For this review, take the finished solid that the model builds, in its own axes (mm). A direction names the side the tool comes from. Round coordinates to 2 decimals unless told otherwise and drop trailing zeros. Order: outer loops, then holes, each group sorted by start corner. A loop starts at its lowest first (then second) coordinate and runs counter-clockwise, first axis right, second up. Notation, with made-up numbers: (36, -18.75) -> (62, -18.75) arc R32 ccw to (62, 9.25) -> close; hole circle Ø3 at (-18, -23.75). An arc over 180 degrees is marked (long way). Answer in a Markdown table with one row per item.
```python
from build123d import *

# Parameters (mm, degrees)
SKETCH1_W           = 55
SKETCH1_H           = 67
BOSS_EXTRUDE1_DEPTH = 60
SKETCH3_W           = 8
SKETCH3_H           = 17.5
CUT_EXTRUDE3_DEPTH  = 58
SKETCH4_W           = 4
SKETCH4_H           = 1
SKETCH4_W_2         = 2.5
SKETCH4_H_2         = 15.5
SKETCH4_W_3         = 8
BOSS_EXTRUDE2_DEPTH = 2


with BuildPart() as part:
    # Sketch1 → Boss-Extrude1 (new body)
    with BuildSketch(Plane(origin=(0, 0, 0), x_dir=(1, 0, 0), z_dir=(0, 1, 0))):
        Rectangle(SKETCH1_W, SKETCH1_H)
    extrude(amount=BOSS_EXTRUDE1_DEPTH)

    # Sketch3 → Cut-Extrude3 (cut)
    with BuildSketch(Plane(origin=(0, 60, 0), x_dir=(1, 0, 0), z_dir=(0, 1, 0))):
        Polygon((-18, 13.5), (-18, 31), (-4, 31), (-4, 13.5), (4, 13.5), (4, 31), (18, 31), (18, 13.5), (25.5, 13.5), (25.5, 0.5), (18, 0.5), (18, -17), (25.5, -17), (25.5, -30), (-25.5, -30), (-25.5, -17), (-18, -17), (-18, 0.5), (-25.5, 0.5), (-25.5, 13.5), align=None)
        with Locations((0, -8.25)):
            Rectangle(SKETCH3_W, SKETCH3_H, mode=Mode.SUBTRACT)
    extrude(amount=-CUT_EXTRUDE3_DEPTH, mode=Mode.SUBTRACT)

    # Sketch4 → Boss-Extrude2 (add)
    with BuildSketch(Plane(origin=(0, 60, 0), x_dir=(1, 0, 0), z_dir=(0, 1, 0))):
        with Locations((-20, 30.5)):
            Rectangle(SKETCH4_W, SKETCH4_H)
        Polygon((4, 31), (-4, 31), (-4, 30), (-1.25, 30), (1.25, 30), (4, 30), align=None)
        with Locations((0, 22.25)):
            Rectangle(SKETCH4_W_2, SKETCH4_H_2)
        with Locations((20, 30.5)):
            Rectangle(SKETCH4_W, SKETCH4_H)
        with Locations((20, 14)):
            Rectangle(SKETCH4_W, SKETCH4_H)
        Polygon((-1.25, 14.5), (-4, 14.5), (-4, 13.5), (4, 13.5), (4, 14.5), (1.25, 14.5), align=None)
        with Locations((-20, 14)):
            Rectangle(SKETCH4_W, SKETCH4_H)
        with Locations((-20, 0)):
            Rectangle(SKETCH4_W, SKETCH4_H)
        Rectangle(SKETCH4_W_3, SKETCH4_H)
        with Locations((20, 0)):
            Rectangle(SKETCH4_W, SKETCH4_H)
        with Locations((20, -16.5)):
            Rectangle(SKETCH4_W, SKETCH4_H)
        with Locations((-20, -16.5)):
            Rectangle(SKETCH4_W, SKETCH4_H)
        with Locations((0, -16.5)):
            Rectangle(SKETCH4_W_3, SKETCH4_H)
        with Locations((0, -8.25)):
            Rectangle(SKETCH4_W_2, SKETCH4_H_2)
    extrude(amount=BOSS_EXTRUDE2_DEPTH)


solid = part.part
```
Q1. Take a section at C-C, the plane z = 28. Write out the cut boundary in (x, y).
Answer key:
| item | result |
|---|---|
| outline | (-27.5, 0) -> (27.5, 0) -> (27.5, 60) -> (25.5, 60) -> (25.5, 2) -> (-25.5, 2) -> (-25.5, 60) -> (-27.5, 60) -> close |
Q2. Take a section at B-B, the plane x = -20.5. Write out the cut boundary in (y, z).
Answer key:
| item | result |
|---|---|
| outline | (0, -33.5) -> (60, -33.5) -> (60, -31) -> (62, -31) -> (62, -30) -> (60, -30) -> (60, -14.5) -> (62, -14.5) -> (62, -13.5) -> (2, -13.5) -> (2, -0.5) -> (62, -0.5) -> (62, 0.5) -> (60, 0.5) -> (60, 16) -> (62, 16) -> (62, 17) -> (2, 17) -> (2, 30) -> (60, 30) -> (60, 33.5) -> (0, 33.5) -> close |
Q3. Take a section at A-A, the plane y = 52. Write out the cut boundary in (x, z), then the cut area to 3 significant figures.
Answer key:
| item | result |
|---|---|
| outline | (-27.5, -33.5) -> (27.5, -33.5) -> (27.5, 33.5) -> (-27.5, 33.5) -> close; (-4, -0.5) -> (4, -0.5) -> (4, 17) -> (-4, 17) -> close; hole (-25.5, -13.5) -> (-18, -13.5) -> (-18, -31) -> (-4, -31) -> (-4, -13.5) -> (4, -13.5) -> (4, -31) -> (18, -31) -> (18, -13.5) -> (25.5, -13.5) -> (25.5, -0.5) -> (18, -0.5) -> (18, 17) -> (25.5, 17) -> (25.5, 30) -> (-25.5, 30) -> (-25.5, 17) -> (-18, 17) -> (-18, -0.5) -> (-25.5, -0.5) -> close |
| area | 1,380 mm^2 |
Q4. Clearance check with flat-ended pins moving along their axes: pin 1 Ø1.4 at (x, z) = (-2.5, -20) entering from +Y; pin 2 Ø1 at (x, z) = (16, 7.5) entering from +Y; pin 3 Ø1 at (x, y) = (-19, 61.5) entering from +Z; pin 4 Ø1.1 at (y, z) = (60.5, 0) entering from +X. State where each tip first meets the part, or that it passes through.
Answer key:
| item | result |
|---|---|
| pin 1 | stops at y = 60 |
| pin 2 | stops at y = 2 |
| pin 3 | stops at z = 17 |
| pin 4 | stops at x = 27.5 |
Q5. Take a section at D-D, the plane z = 13.5. Write out the cut boundary in (x, y).
Answer key:
| item | result |
|---|---|
| outline | (-27.5, 0) -> (27.5, 0) -> (27.5, 60) -> (18, 60) -> (18, 2) -> (4, 2) -> (4, 60) -> (1.25, 60) -> (1.25, 62) -> (-1.25, 62) -> (-1.25, 60) -> (-4, 60) -> (-4, 2) -> (-18, 2) -> (-18, 60) -> (-27.5, 60) -> close |
Q6. Tool access review of faces 1 (the face through (-18, 32, 8)), 2 (the face through (0, 0, 0)), 3 (the face through (0, 61, -31)), 4 (the face through (-1.25, 61, 8)), 5 (the face through (3, 61, -14.5)): name each direction out of +Z, -Z, +X, -X, +Y, -Y from which nothing blocks a thin tool from reaching the whole face with its end or side.
Answer key:
| item | result |
|---|---|
| face 1 | +Y |
| face 2 | +Z, -Z, +X, -X, -Y |
| face 3 | -Z, +X, -X, +Y |
| face 4 | -X, +Y |
| face 5 | +X, +Y |
Q7. To check wall thickness, follow probe 1 along X at (y, z) = (42, 9.5); probe 2 along Z at (x, y) = (18.5, 5.5); probe 3 along X at (y, z) = (39, -11.5). State the ranges of each line that lie inside material, in increasing order.
Answer key:
| item | result |
|---|---|
| probe 1 | x = -27.5 to -18, -4 to 4, 18 to 27.5 |
| probe 2 | z = -33.5 to -13.5, -0.5 to 17, 30 to 33.5 |
| probe 3 | x = -27.5 to -25.5, 25.5 to 27.5 |
Q8. The part is to be moulded in two halves that separate along X. For faces 6 (the face through (-25.5, 31, 24)), 7 (the face through (3, 60, -22)), 8 (the face through (1.25, 61, 8)), say which applies: +X half, -X half, draft (parallel to the pull), parting line (faces both ways), or undercut.
Answer key:
| item | result |
|---|---|
| face 6 | undercut |
| face 7 | draft |
| face 8 | +X half |
